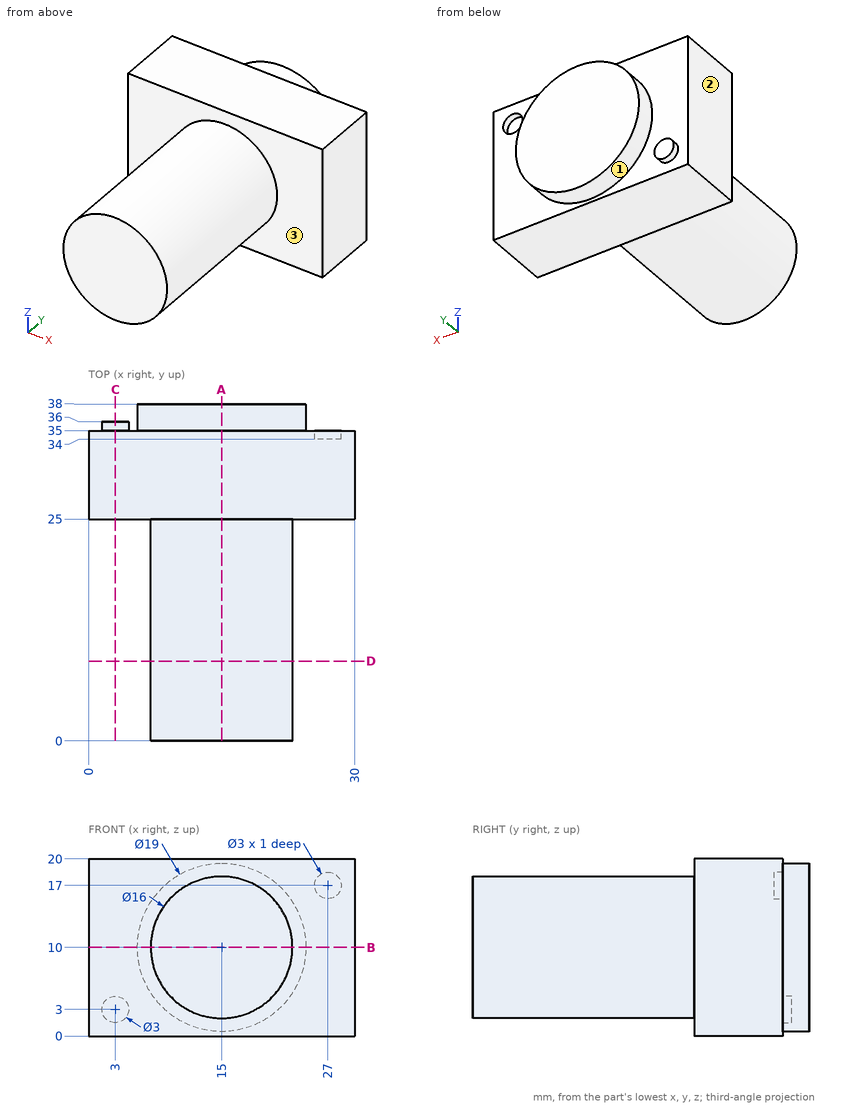
For this review, use the dimensioned drawing (mm, ordinates from the lowest corner) and the shaded views. A direction names the side the tool comes from. Give positions to 0.01 mm unless a question says otherwise; leave off trailing zeros. Write each loop counter-clockwise with the first axis right and the second up, starting at its lowest first coordinate (ties: lowest second). Pieces come first, ordered by that corner, then holes. Notation, with made-up numbers: M 34,22.5 L 75,22.5 A18 cw 75,42.5 Z; hole C -11,75.5 d9. An arc over 180 degrees is marked long. Answer as a JSON object with one key per item and string values. Group by question number.
1) Tool access review of the marked faces 1, 2 and 3: name each direction out of +Z, -Z, +X, -X, +Y, -Y from which nothing blocks a thin tool from reaching the whole face with its end or side.
2) We need section D-D (y = 9). Give the boundary of the cut face in (x, z), and give its area (3 significant figures).
3) Clearance check with flat-ended pins moving along their axes: pin 1 Ø2 at (x, y) = (7, 13.5) entering from +Z; pin 2 Ø4 at (x, z) = (27, 17) entering from -Y; pin 3 Ø0.9 at (x, z) = (26.5, 17.5) entering from +Y; pin 4 Ø5 at (x, z) = (21, 11) entering from -Y. State where each tip first meets the part, or that it passes through.
4) We need section B-B (z = 10). Give the boundary of the cut face in (x, y).
5) We need section A-A (x = 15). Give the boundary of the cut face in (y, z), and give its area (3 significant figures).
6) For line 1 along X through (y, z) = (34.35, 17); line 2 along Y through (x, z) = (25, 8.5); line 3 along Y through (x, z) = (21.5, 15), list the stretches that pass through material, from the lowest coordinate up.
7) We need section C-C (x = 3). Give the boundary of the cut face in (y, z), and give its area (3 significant figures).
Answer key:
{
 "1": {"face 1": "+Y", "face 2": "+Z, -Z, -X, +Y, -Y", "face 3": "-Y"},
 "2": {"outline": "C 15,10 d16", "area": "201 mm²"},
 "3": {"pin 1": "stops at z = 13.87", "pin 2": "stops at y = 25", "pin 3": "stops at y = 34", "pin 4": "stops at y = 0"},
 "4": {"outline": "M 0,25 L 7,25 L 7,0 L 23,0 L 23,25 L 30,25 L 30,35 L 24.5,35 L 24.5,38 L 5.5,38 L 5.5,35 L 0,35 Z"},
 "5": {"outline": "M 0,2 L 25,2 L 25,0 L 35,0 L 35,0.5 L 38,0.5 L 38,19.5 L 35,19.5 L 35,20 L 25,20 L 25,18 L 0,18 Z", "area": "657 mm²"},
 "6": {"line 1": "x = 0 to 25.5, 28.5 to 30", "line 2": "y = 25 to 35", "line 3": "y = 25 to 38"},
 "7": {"outline": "M 25,0 L 35,0 L 35,1.5 L 36,1.5 L 36,4.5 L 35,4.5 L 35,20 L 25,20 Z", "area": "203 mm²"}
}
